Work out the finished part from the listing and answer in its coordinate system (mm). Coordinates: 2 decimals unless noted, no trailing zeros. Order: outer loops, then holes, each group sorted by start corner. A loop starts at its lowest first (then second) coordinate and runs counter-clockwise, first axis right, second up. Notation, with made-up numbers: (17, 37) - (39, 37) arc R32 cw to (39, 70) - close; hole circle Ø7 at (26, 63.25). An arc over 180 degrees is marked (long way). Answer as a JSON object with one key per item and string values. Group by question number.
1) Each of these flat-tipped pins is pushed along its axis until it touches: P1, Ø2.5, axis at x = 5, z = -48.5, coming from the -Y side; P2, Ø1.9, axis at x = 2, y = 3, coming from the +Z side; P3, Ø0.7, axis at x = 2.5, z = -94.5, coming from the +Y side. Where does it stop, or does it pass through?
2) Find the intervals of material crossed by line 1 along Z through (x, y) = (5.5, 374.5); line 2 along Z through (x, y) = (5.5, 275); line 3 along Z through (x, y) = (3.75, 446), in increasing order.
3) Section B-B (x = 2.5) is taken. Count the separate pieces of the cut face and the enclosed holes in it, plus the area to 3 significant figures.
4) Section A-A (y = 76) is taken. Give the vertices of the cut face in (x, z), plus the area to 3 significant figures.
5) The mould has two halves that part along Z. Classify faces 1 (the face through (0, 201, -186)), 2 (the face through (3.13, 276.14, -96.58)), 3 (the face through (3.1, 361.1, -158.4)): released by +Z, released by -Z, zero draft, split by the parting line, or undercut.
from build123d import *

# Parameters (mm, degrees)
BOSS_EXTRUDE1_DEPTH = 6.35
CUT_EXTRUDE1_DEPTH  = 6.35
SKETCH5_R           = 2
SKETCH5_W           = 6.35
SKETCH5_H           = 12.7
SKETCH5_W_2         = 12.7
SKETCH5_H_2         = 6.35
CUT_EXTRUDE2_DEPTH  = 6.35
SKETCH6_W           = 6.35
SKETCH6_H           = 12.7
CUT_EXTRUDE3_DEPTH  = 6.35
SKETCH7_W           = 12.7
SKETCH7_H           = 6.35
CUT_EXTRUDE4_DEPTH  = 6.35


with BuildPart() as part:
    # Sketch1 → Boss-Extrude1 (new body)
    with BuildSketch(Plane(origin=(0, 0, 0), x_dir=(0, 0, -1), z_dir=(1, 0, 0))):
        Polygon((12.7, 6.35), (12.7, 0), (25.4, 0), (25.4, 6.35), (63.5, 6.35), (63.5, 0), (76.2, 0), (76.2, 6.35), (120.65, 6.35), (120.65, 0), (133.35, 0), (133.35, 6.35), (146.05, 6.35), (146.05, 0), (158.75, 0), (158.75, 6.35), (171.45, 6.35), (171.45, 0), (176.749457482, 0), (184.15, 0), (184.15, 6.35), (196.85, 6.35), (196.85, 0), (260.35, 0), (260.35, 508), (190.5, 508), (0, 37.703125), (0, 6.35), align=None)
        Polygon((133.35, 299.255680579), (184.15, 424.668180579), (184.15, 69.85), (133.35, 69.85), (133.35, 274.095300459), align=None, mode=Mode.SUBTRACT)
    extrude(amount=BOSS_EXTRUDE1_DEPTH)

    # Sketch3 → Cut-Extrude1 (cut)
    with BuildSketch(Plane(origin=(6.35, 0, 0), x_dir=(0, 0, -1), z_dir=(1, 0, 0))):
        Polygon((49.2125, 17.4625), (49.2125, 14.2875), (46.83125, 14.2875), (46.83125, 6.35), (42.06875, 6.35), (42.06875, 14.2875), (39.6875, 14.2875), (39.6875, 17.4625), (42.06875, 17.4625), (42.06875, 20.6375), (46.83125, 20.6375), (46.83125, 17.4625), align=None)
        Polygon((103.1875, 17.4625), (103.1875, 14.2875), (100.80625, 14.2875), (100.80625, 6.35), (96.04375, 6.35), (96.04375, 14.2875), (93.6625, 14.2875), (93.6625, 17.4625), (96.04375, 17.4625), (96.04375, 20.6375), (100.80625, 20.6375), (100.80625, 17.4625), align=None)
    extrude(amount=-CUT_EXTRUDE1_DEPTH, mode=Mode.SUBTRACT)

    # Sketch5 → Cut-Extrude2 (cut)
    with BuildSketch(Plane(origin=(6.35, 0, 0), x_dir=(0, 0, -1), z_dir=(1, 0, 0))):
        with Locations((193.675, 127)):
            Circle(SKETCH5_R)
        with Locations((193.675, 381)):
            Circle(SKETCH5_R)
        with Locations((193.675, 57.15)):
            Rectangle(SKETCH5_W, SKETCH5_H)
        with Locations((193.675, 196.85)):
            Rectangle(SKETCH5_W, SKETCH5_H)
        with Locations((241.3, 371.475)):
            Rectangle(SKETCH5_W_2, SKETCH5_H_2)
        with Locations((241.3, 123.825)):
            Rectangle(SKETCH5_W_2, SKETCH5_H_2)
        with Locations((241.3, 136.525)):
            Rectangle(SKETCH5_W_2, SKETCH5_H_2)
        with Locations((241.3, 384.175)):
            Rectangle(SKETCH5_W_2, SKETCH5_H_2)
        with Locations((193.675, 311.15)):
            Rectangle(SKETCH5_W, SKETCH5_H)
        with Locations((193.675, 450.85)):
            Rectangle(SKETCH5_W, SKETCH5_H)
    extrude(amount=-CUT_EXTRUDE2_DEPTH, mode=Mode.SUBTRACT)

    # Sketch6 → Cut-Extrude3 (cut)
    with BuildSketch(Plane(origin=(6.35, 0, 0), x_dir=(0, 0, -1), z_dir=(1, 0, 0))):
        with Locations((123.825, 44.45)):
            Rectangle(SKETCH6_W, SKETCH6_H)
    extrude(amount=-CUT_EXTRUDE3_DEPTH, mode=Mode.SUBTRACT)

    # Sketch7 → Cut-Extrude4 (cut)
    with BuildSketch(Plane(origin=(6.35, 0, 0), x_dir=(0, 0, -1), z_dir=(1, 0, 0))):
        with Locations((241.3, 219.075)):
            Rectangle(SKETCH7_W, SKETCH7_H)
    extrude(amount=-CUT_EXTRUDE4_DEPTH, mode=Mode.SUBTRACT)


solid = part.part
Report:
{
 "1": {"P1": "stops at y = 6.35", "P2": "stops at z = -12.7", "P3": "stops at y = 271.86"},
 "2": {"line 1": "z = -260.35 to -247.65, -234.95 to -184.15, -163.83 to -136.42", "line 2": "z = -260.35 to -184.15, -133.35 to -96.12", "line 3": "z = -260.35 to -196.85, -190.5 to -165.39"},
 "3": {"separate pieces": "1", "enclosed holes": "13", "area": "70,800 mm²"},
 "4": {"outline": "(0, -260.35) - (6.35, -260.35) - (6.35, -184.15) - (0, -184.15) - close; (0, -133.35) - (6.35, -133.35) - (6.35, -15.51) - (0, -15.51) - close", "area": "1,230 mm²"},
 "5": {"face 1": "zero draft", "face 2": "released by +Z", "face 3": "undercut"}
}
